Geometry: final body of the model. Coordinates: model frame, mm. Give positions to 0.01 mm unless a question says otherwise; leave off trailing zeros. Order: outer loops, then holes, each group sorted by start corner. A loop starts at its lowest first (then second) coordinate and runs counter-clockwise, first axis right, second up. Notation, with made-up numbers: (42, 43.5) -> (72, 43.5) arc R34 cw to (72, 77.5) -> close; hole circle Ø6 at (-19.5, 3.5). An arc over 180 degrees is marked (long way). Write item = value, one per line.
```python
from build123d import *

# Parameters (mm, degrees)
SKETCH_2_W            = 200
SKETCH_2_H            = 208
EXTRUDE_1_DEPTH       = 5
HOLE_WIZARD_4_0_4_1_D = 4
HOLE_WIZARD_5_0_5_1_D = 5


with BuildPart() as part:
    # 草图2 → 凸台-拉伸1 (new body)
    with BuildSketch(Plane(origin=(0, 0, 0), x_dir=(1, 0, 0), z_dir=(0, 1, 0))):
        with Locations((100, 104)):
            Rectangle(SKETCH_2_W, SKETCH_2_H)
    extrude(amount=EXTRUDE_1_DEPTH)

    # Ø4.0 (4) 直径孔1 (through all)
    with Locations(Plane(origin=(0, 5, 0), x_dir=(1, 0, 0), z_dir=(0, 1, 0))):
        with Locations((60, 168), (85, 168), (60, 138), (85, 138), (60, 60), (85, 60), (60, 30), (85, 30), (115, 30), (140, 30), (115, 60), (140, 60), (115, 138), (140, 138), (115, 168), (140, 168)):
            Hole(HOLE_WIZARD_4_0_4_1_D / 2)

    # Ø5.0 (5) 直径孔1 (through all)
    with Locations(Plane(origin=(0, 5, 0), x_dir=(1, 0, 0), z_dir=(0, 1, 0))):
        with Locations((10, 168), (10, 138), (10, 60), (10, 30), (70, 198), (70, 10), (130, 10), (130, 198), (190, 30), (190, 60), (190, 138), (190, 168)):
            Hole(HOLE_WIZARD_5_0_5_1_D / 2)


solid = part.part
```
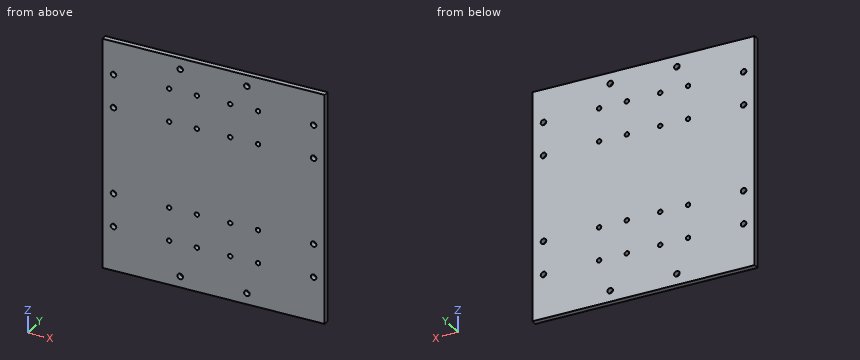
1) Section query B-B (z = -198). Output: boundary loops of the cut face in (x, y).
Check sheet entries:
outline = (0, 0) -> (67.5, 0) -> (67.5, 5) -> (0, 5) -> close; (72.5, 0) -> (127.5, 0) -> (127.5, 5) -> (72.5, 5) -> close; (132.5, 0) -> (200, 0) -> (200, 5) -> (132.5, 5) -> close
2) Section query C-C (x = 190). Output: boundary loops of the cut face in (y, z), plus the area to 3 significant figures.
Check sheet entries:
outline = (0, -208) -> (5, -208) -> (5, -170.5) -> (0, -170.5) -> close; (0, -165.5) -> (5, -165.5) -> (5, -140.5) -> (0, -140.5) -> close; (0, -135.5) -> (5, -135.5) -> (5, -62.5) -> (0, -62.5) -> close; (0, -57.5) -> (5, -57.5) -> (5, -32.5) -> (0, -32.5) -> close; (0, -27.5) -> (5, -27.5) -> (5, 0) -> (0, 0) -> close
area = 940 mm²
3) Line query: line 1 (Z direction, x = 115, y = 2); line 2 (Z direction, x = 70, y = 1); line 3 (Z direction, x = 190, y = 2.2). Output: solid intervals per line, ascending. Write a range as from..to.
Check sheet entries:
line_1 = -208..-170, -166..-140, -136..-62, -58..-32, -28..0
line_2 = -208..-200.5, -195.5..-12.5, -7.5..0
line_3 = -208..-170.5, -165.5..-140.5, -135.5..-62.5, -57.5..-32.5, -27.5..0
4) Section query A-A (x = 70). Output: boundary loops of the cut face in (y, z).
Check sheet entries:
outline = (0, -208) -> (5, -208) -> (5, -200.5) -> (0, -200.5) -> close; (0, -195.5) -> (5, -195.5) -> (5, -12.5) -> (0, -12.5) -> close; (0, -7.5) -> (5, -7.5) -> (5, 0) -> (0, 0) -> close
